For this review, take the finished solid that the model builds, in its own axes (mm). Face numbers are marked on the shaded views. Coordinates: 2 decimals unless noted, no trailing zeros. Write each loop counter-clockwise with the first axis right and the second up, starting at its lowest first coordinate (ties: lowest second). Pieces come first, ordered by that corner, then holes. Notation, with made-up numbers: (41, 1.25) -> (71, 1.25) arc R30 cw to (71, 25.25) -> close; hole circle Ø6 at (88.25, 39.5). An arc over 180 degrees is marked (long way). One line per item, written item: value. Start each with the question number.
1) Add section D-D (y = 8). State the section outline as (x, z) points, and give its area (3 significant figures).
2) Mouldability with a two-part tool opening along Y and no side actions: class the marked faces 1, 2 and 3 as released by +Y, released by -Y, zero draft, split by the parting line, or undercut.
3) For probe 1 along Y at (x, z) = (0, 31.5); probe 2 along Y at (x, z) = (0, 79.25); probe 3 along Z at (x, y) = (6, 5.5), list the stretches that pass through material, from the lowest coordinate up. Write a range as from..to.
4) Add section A-A (x = 0). State the section outline as (y, z) points, and give its area (3 significant figures).
5) Add section C-C (z = 73.5). State the section outline as (x, y) points.
6) For pin 1 Ø6 at (x, z) = (-5.5, 67.5) entering from +Y; pin 2 Ø4 at (y, z) = (5.5, 11.5) entering from +X; pin 3 Ø12 at (x, y) = (7, -6.5) entering from -Z; pin 4 Ø3 at (x, z) = (7, 11.5) entering from -Y, all flat-tipped, find the tip position at first contact; note any pin that passes through.
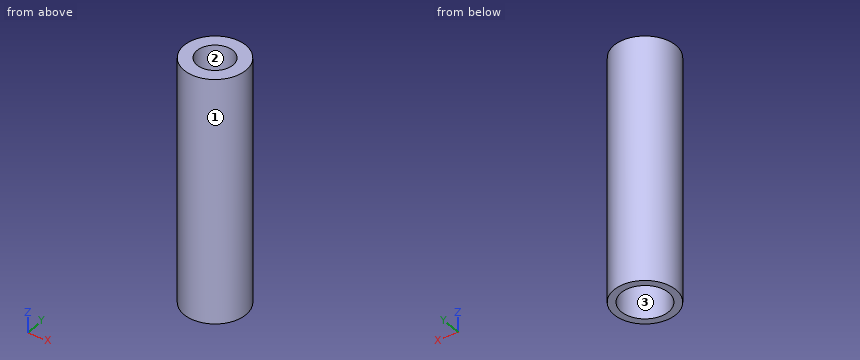
from build123d import *

# Parameters (mm, degrees)
CYLINDER_R           = 12
CYLINDER_DEPTH       = 95
SKETCH_R             = 9.2
POCKET_DEPTH         = 70
SKETCH001_R          = 7
POCKET001_DEPTH      = 0.001
POCKET001_DEPTH_BACK = -95.001


with BuildPart() as part:
    # Cylinder → Cylinder (new body)
    with BuildSketch(Plane.XY):
        Circle(CYLINDER_R)
    extrude(amount=CYLINDER_DEPTH)

    # Sketch → Pocket (cut)
    with BuildSketch(Plane.XY):
        Circle(SKETCH_R)
    extrude(amount=POCKET_DEPTH, mode=Mode.SUBTRACT)

    # Sketch001 → Pocket001 (cut, two sides)
    with BuildSketch(Plane.XY) as pocket001_sk:
        Circle(SKETCH001_R)
    extrude(amount=-POCKET001_DEPTH, mode=Mode.SUBTRACT)
    extrude(pocket001_sk.sketch, amount=-POCKET001_DEPTH_BACK, mode=Mode.SUBTRACT)


solid = part.part
Numbers:
1. outline: (-8.94, 0) -> (-4.54, 0) -> (-4.54, 70) -> (4.54, 70) -> (4.54, 0) -> (8.94, 0) -> (8.94, 95) -> (-8.94, 95) -> close
1. area: 1,060 mm²
2. face 1: split by the parting line
2. face 2: undercut
2. face 3: undercut
3. probe 1: -12..-9.2, 9.2..12
3. probe 2: -12..-7, 7..12
3. probe 3: 70..95
4. outline: (-12, 0) -> (-9.2, 0) -> (-9.2, 70) -> (-7, 70) -> (-7, 95) -> (-12, 95) -> close; (7, 70) -> (9.2, 70) -> (9.2, 0) -> (12, 0) -> (12, 95) -> (7, 95) -> close
4. area: 642 mm²
5. outline: circle Ø24 at (0, 0); hole circle Ø14 at (0, 0)
6. pin 1: y = 11.74
6. pin 2: x = 11.48
6. pin 3: z = 0
6. pin 4: y = -10.67
